Geometry: final body of the model. Coordinates: model frame, mm. Face numbers are marked on the shaded views. A direction names the side the tool comes from. Coordinates: 2 decimals unless noted, no trailing zeros. Write each loop counter-clockwise with the first axis right and the second up, starting at its lowest first coordinate (ties: lowest second). Pieces come first, ordered by that corner, then holes. Notation, with made-up numbers: (-6, -15.5) - (-1, -15.5) arc R20 ccw to (-1, -1.5) - close; hole circle Ø3 at (80.5, -29). An arc over 180 degrees is marked (long way). Answer as a JSON object with one key per item and string values. Group by question number.
Item 1: Section A-A on y = 0. Return loops of the section in (x, z).
Item 2: Mould query, pull axis Z, two halves, no side actions, for the marked faces 5, 6, 7 and 8. Classes: pulls with the +Z half, pulls with the -Z half, needs draft (parallel to the pull), parting line crosses it, or undercut.
Item 3: First-contact query: pin 1 Ø2 at (x, z) = (-2.5, -3) entering from -Y; pin 2 Ø1.5 at (x, y) = (-3.5, 3) entering from +Z; pin 3 Ø1.9 at (x, y) = (-1.5, 0) entering from -Z. Flat tips, straight axial feed; report the tip coordinate or a pass-through.
Item 4: Set-up query: the marked faces 1, 2, 3 and 4. Return all of +Z, -Z, +X, -X, +Y, -Y with unobstructed straight access to the full face (end or side cutting, diameter ignored); none if empty.
Item 5: Line query: line 1 along X through (y, z) = (4.25, 2.5); line 2 along Z through (x, y) = (0.5, 0); line 3 along Y through (x, z) = (-1, 0). Output: solid intervals per line, ascending. Write a range as from..to.
Item 6: Section B-B on z = 0. Return loops of the section in (x, y).
Item 7: Section C-C on z = 5.75. Return loops of the section in (x, y), and give its area (3 significant figures).
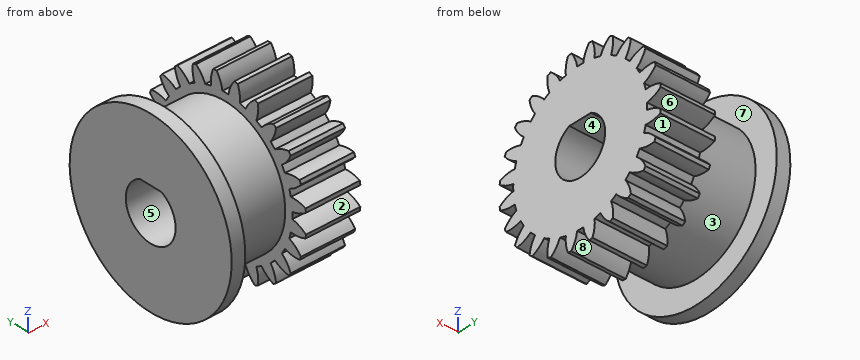
```python
from build123d import *

# Parameters (mm, degrees)
BASPROSKE_W         = 4
BASPROSKE_H         = 6.5
TOOTHCUT_DEPTH      = 11.024968828
TEETHCUTS_COUNT     = 24
TEETHCUTS_ANGLE     = 345
BORSKE_R            = 1.5
BORE_DEPTH          = 50.0000508
SKETCH_1_R          = 4.8
SKETCH_1_R_2        = 1.5
EXTRUDE_1_DEPTH     = 4.5
SKETCH_2_R          = 6.5
SKETCH_2_R_2        = 1.5
EXTRUDE_2_DEPTH     = 1
CUT_EXTRUDE_1_REACH = 15.219


with BuildPart() as part:
    # BasProSke → Base-Revolve (revolve)
    with BuildSketch(Plane(origin=(0, 0, 0), x_dir=(1, 0, 0), z_dir=(0, 1, 0)), mode=Mode.PRIVATE) as base_revolve_sk:
        with Locations((2, 3.25)):
            Rectangle(BASPROSKE_W, BASPROSKE_H)
    revolve(base_revolve_sk.sketch.rotate(Axis((-10, 0, 0), (1, 0, 0)), 180), axis=Axis((-10, 0, 0), (1, 0, 0)))

    # TooCutSke → ToothCut (cut, through all)
    with BuildSketch(Plane(origin=(0, 0, 0), x_dir=(0, 0, -1), z_dir=(1, 0, 0))):
        with BuildLine():
            ThreePointArc((0.241646108, 5.368564348), (0, 5.374), (-0.241646108, 5.368564348))
            ThreePointArc((-0.241646108, 5.368564348), (-0.413699957, 5.957993365), (-0.729686037, 6.48447403))
            ThreePointArc((-0.729686037, 6.48447403), (0, 6.5254), (0.729686037, 6.48447403))
            ThreePointArc((0.729686037, 6.48447403), (0.413699957, 5.957993365), (0.241646108, 5.368564348))
        make_face()
    toothcut = extrude(amount=TOOTHCUT_DEPTH, mode=Mode.SUBTRACT)

    # TeethCuts: ToothCut ×24 about axis
    teethcuts_axis = Axis((-10, 0, 0), (1, 0, 0))
    for i in range(1, TEETHCUTS_COUNT):
        add(toothcut.rotate(teethcuts_axis, i * TEETHCUTS_ANGLE / (TEETHCUTS_COUNT - 1)), mode=Mode.SUBTRACT)

    # BorSke → Bore (cut, symmetric)
    with BuildSketch(Plane(origin=(0, 0, 0), x_dir=(0, 0, -1), z_dir=(1, 0, 0))):
        with Locations(Location((0, 0, 0), (0, 0, 180))):
            Circle(BORSKE_R)
    extrude(amount=BORE_DEPTH, both=True, mode=Mode.SUBTRACT)

    # 草图1 → 凸台-拉伸1 (add)
    with BuildSketch(Plane.ZY):
        with Locations(Location((0, 0, 0), (0, 0, 180))):
            Circle(SKETCH_1_R)
        Circle(SKETCH_1_R_2, mode=Mode.SUBTRACT)
    extrude(amount=EXTRUDE_1_DEPTH)

    # 草图2 → 凸台-拉伸2 (add)
    with BuildSketch(Plane.ZY.offset(4.5)):
        Circle(SKETCH_2_R)
        Circle(SKETCH_2_R_2, mode=Mode.SUBTRACT)
    extrude(amount=EXTRUDE_2_DEPTH)

    # 草图3 → 切除-拉伸1 (cut, up to next)
    with BuildSketch(Plane.ZY.offset(5.5), mode=Mode.PRIVATE) as cut_extrude_1_sk1:
        with BuildLine():
            Line((1.8, -0.871779789), (1.8, 0.871779789))
            ThreePointArc((1.8, 0.871779789), (-2, 0), (1.8, -0.871779789))
        make_face()
    cut_extrude_1_tool1 = extrude(cut_extrude_1_sk1.sketch, amount=-CUT_EXTRUDE_1_REACH, mode=Mode.PRIVATE) & part.part
    add(cut_extrude_1_tool1.solids().sort_by_distance((-5.5, 0, -0.035819))[0], mode=Mode.SUBTRACT)


solid = part.part
```
Checks:
{
 "1": {"outline": "(-5.5, -6.5) - (-4.5, -6.5) - (-4.5, -4.8) - (0, -4.8) - (0, -5.37) - (4, -5.37) - (4, -2) - (-5.5, -2) - close; (-5.5, 1.8) - (4, 1.8) - (4, 5.37) - (0, 5.37) - (0, 4.8) - (-4.5, 4.8) - (-4.5, 6.5) - (-5.5, 6.5) - close"},
 "2": {"face 5": "undercut", "face 6": "undercut", "face 7": "needs draft", "face 8": "pulls with the -Z half"},
 "3": {"pin 1": "y = -4.36", "pin 2": "z = 4.24", "pin 3": "z = -4.8"},
 "4": {"face 1": "+X", "face 2": "+X, -Y", "face 3": "none", "face 4": "+X, -X"},
 "5": {"line 1": "-5.5..-4.5, 0..4", "line 2": "-5.37..-2, 1.8..5.37", "line 3": "-4.8..-2, 2..4.8"},
 "6": {"outline": "(-5.5, -6.5) - (-4.5, -6.5) - (-4.5, -4.8) - (0, -4.8) - (0, -5.37) - (4, -5.37) - (4, -2) - (-5.5, -2) - close; (-5.5, 2) - (4, 2) - (4, 5.37) - (0, 5.37) - (0, 4.8) - (-4.5, 4.8) - (-4.5, 6.5) - (-5.5, 6.5) - close"},
 "7": {"outline": "(-5.5, -3.03) - (-4.5, -3.03) - (-4.5, 3.03) - (-5.5, 3.03) - close; (0, -2.63) - (4, -2.63) - (4, -2.03) - (0, -2.03) - close; (0, -1.16) - (4, -1.16) - (4, -0.33) - (0, -0.33) - close; (0, 0.33) - (4, 0.33) - (4, 1.16) - (0, 1.16) - close; (0, 2.03) - (4, 2.03) - (4, 2.63) - (0, 2.63) - close", "area": "17.5 mm^2"}
}
